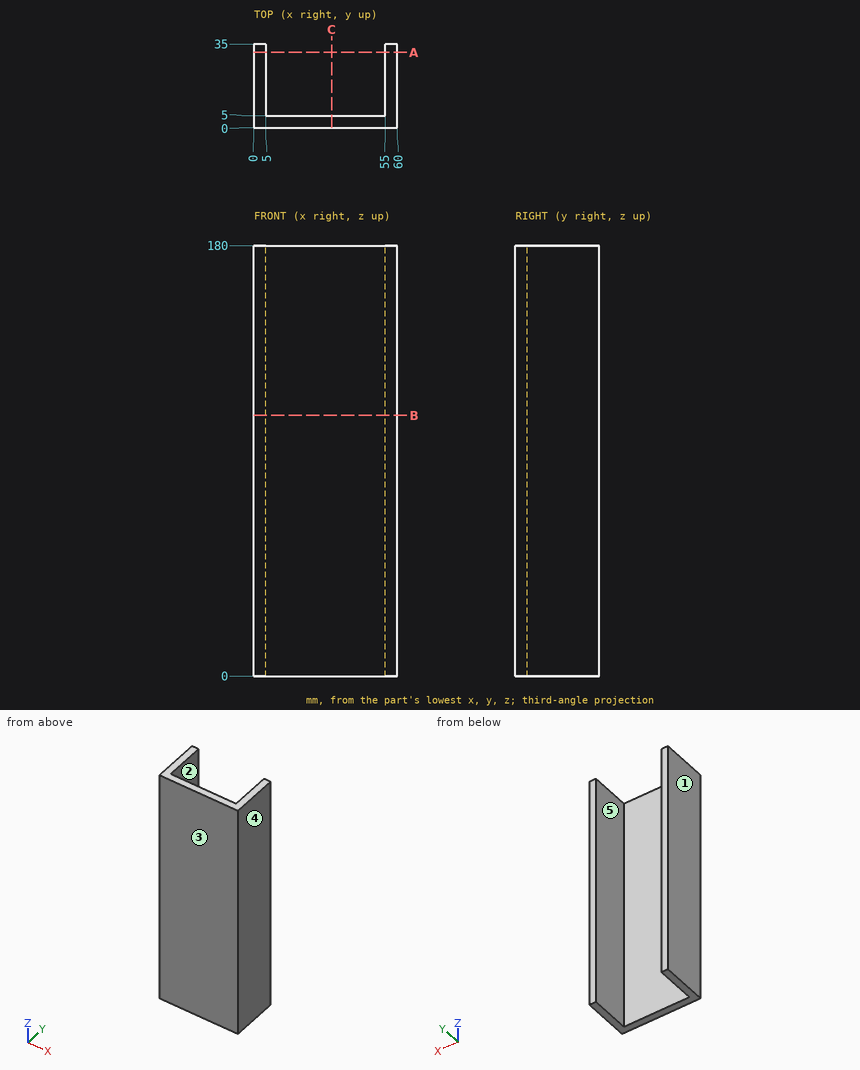
Design review of the part shown in the three views and the two pictorial views. Dimensions are in mm from the part's minimum x, y and z. A direction names the side the tool comes from. Coordinates: 2 decimals unless noted, no trailing zeros. Order: outer loops, then holes, each group sorted by start corner. A loop starts at its lowest first (then second) coordinate and runs counter-clockwise, first axis right, second up.
1) Clearance check with flat-ended pins moving along their axes: pin 1 (15 mm diameter, centred on x = 34.5, z = 130.5, fed in from +Y); pin 2 (3 mm diameter, centred on y = 30.5, z = 154, fed in from -X). State where each tip first meets the part, or that it passes through.
2) Take a section at B-B, the plane z = 109. Give the boundary of the cut face in (x, y), and give its area (3 significant figures).
3) For the marked faces 1 and 2, list the 3-axis set-ups (+Z, -Z, +X, -X, +Y, -Y) from which the entire face can be reached by the end or side of a thin tool; tool diameter is ignored.
4) Wall thickness on line 1 along X through (y, z) = (13.5, 32.5); line 2 along Y through (x, z) = (40, 164): over which ranges is each line inside the solid? List them lowest first.
5) Mouldability with a two-part tool opening along X and no side actions: class the marked faces 3, 4 and 5 as +X half, -X half, draft (parallel to the pull), parting line (faces both ways), or undercut.
6) Take a section at A-A, the plane y = 31.5. Give the boundary of the cut face in (x, z), and give its area (3 significant figures).
7) Take a section at C-C, the plane x = 32.5. Give the boundary of the cut face in (y, z).
Returned:
1. pin 1: stops at y = 5
1. pin 2: stops at x = 0
2. outline: (0, 0) - (60, 0) - (60, 35) - (55, 35) - (55, 5) - (5, 5) - (5, 35) - (0, 35) - close
2. area: 600 mm2
3. face 1: +Z, -Z, -X, +Y, -Y
3. face 2: +Z, -Z, +Y
4. line 1: x = 0 to 5, 55 to 60
4. line 2: y = 0 to 5
5. face 3: draft
5. face 4: +X half
5. face 5: undercut
6. outline: (0, 0) - (5, 0) - (5, 180) - (0, 180) - close; (55, 0) - (60, 0) - (60, 180) - (55, 180) - close
6. area: 1,800 mm2
7. outline: (0, 0) - (5, 0) - (5, 180) - (0, 180) - close
